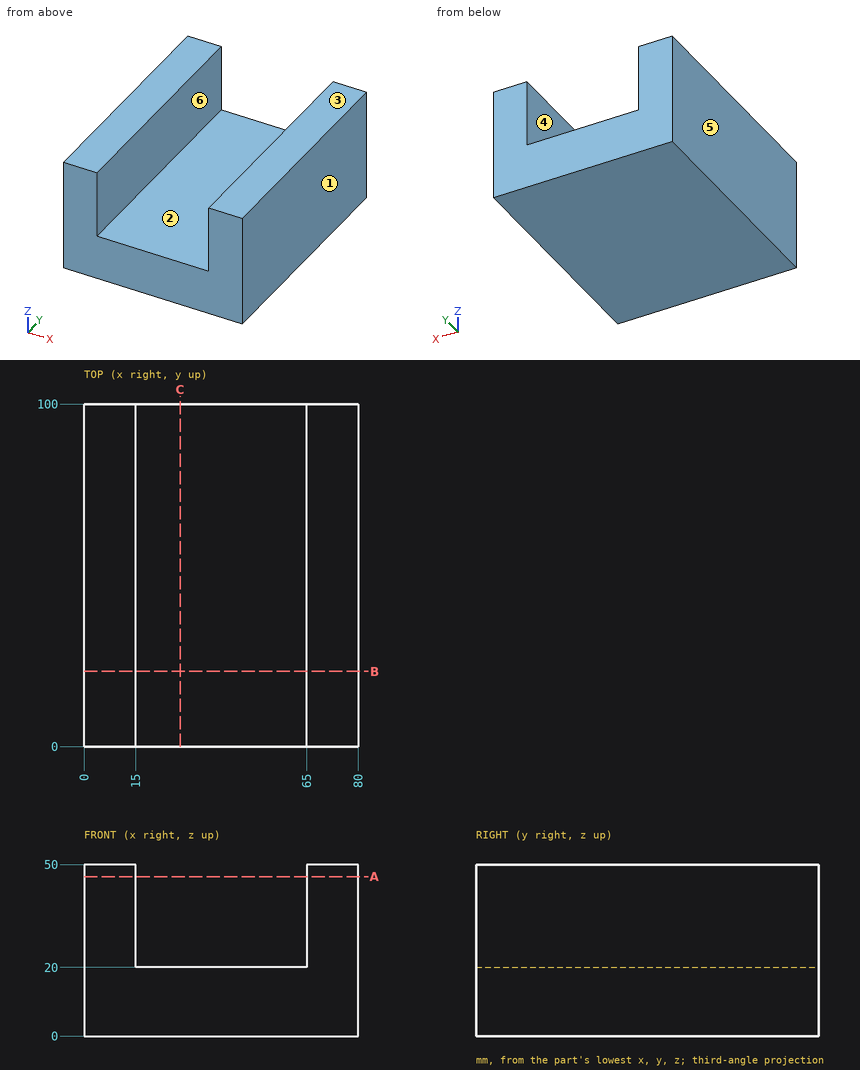
Design review of the part shown in the three views and the two pictorial views. Dimensions are in mm from the part's minimum x, y and z. A direction names the side the tool comes from. Round coordinates to 2 decimals unless told otherwise and drop trailing zeros. Loops run counter-clockwise (first coordinate to the right, second up) from the corner with the lowest first, then second, coordinate; pieces in that order, holes last. Notation, with made-up numbers: (27.5, 79) - (48.5, 79) arc R23 ccw to (48.5, 116) - close; hole circle Ø7 at (22.5, 47.25). An arc over 180 degrees is marked (long way). One line per item, written item: value. Start each with the question number.
Item 1: Take a section at C-C (x = 28). Give the boundary of the cut face in (y, z).
Item 2: For L1, parallel to X at y = 22.5, z = 47.5; L2, parallel to Z at x = 34, y = 41.5, list the stretches that pass through material, from the lowest coordinate up.
Item 3: The part is to be moulded in two halves that separate along X. For the marked faces 3, 4, 5 and 6, say which applies: +X half, -X half, draft (parallel to the pull), parting line (faces both ways), or undercut.
Item 4: For the marked faces 1 and 2, list the 3-axis set-ups (+Z, -Z, +X, -X, +Y, -Y) from which the entire face can be reached by the end or side of a thin tool; tool diameter is ignored.
Item 5: Clearance check with a flat-ended pin moving along its axis: pin 1 Ø3 at (x, y) = (32, 50) entering from +Z. State where the tip first meets the part, or that it passes through.
Item 6: Take a section at B-B (y = 22). Give the boundary of the cut face in (x, z).
Item 7: Take a section at A-A (z = 46.5). Give the boundary of the cut face in (x, y), plus the area to 3 significant figures.
Answer below:
1. outline: (0, 0) - (100, 0) - (100, 20) - (0, 20) - close
2. L1: x = 0 to 15, 65 to 80
2. L2: z = 0 to 20
3. face 3: draft
3. face 4: undercut
3. face 5: -X half
3. face 6: undercut
4. face 1: +Z, -Z, +X, +Y, -Y
4. face 2: +Z, +Y, -Y
5. pin 1: stops at z = 20
6. outline: (0, 0) - (80, 0) - (80, 50) - (65, 50) - (65, 20) - (15, 20) - (15, 50) - (0, 50) - close
7. outline: (0, 0) - (15, 0) - (15, 100) - (0, 100) - close; (65, 0) - (80, 0) - (80, 100) - (65, 100) - close
7. area: 3,000 mm2
